from build123d import *

# Parameters (mm, degrees)
SKETCH_1_W               = 45
SKETCH_1_H               = 45
EXTRUDE_1_DEPTH          = 2.5
EXTRUDE_2_DEPTH          = 50
SKETCH_3_R               = 5.5
CUT_EXTRUDE_1_DEPTH      = 80.633535649
CUT_EXTRUDE_2_DEPTH      = 80.633535649
SKETCH_5_W               = 5
SKETCH_5_H               = 39.075696326
EXTRUDE_3_DEPTH          = 10
CUT_EXTRUDE_3_DEPTH      = 81.922374398
SKETCH_7_W               = 5.5
SKETCH_7_H               = 39.075696326
EXTRUDE_4_DEPTH          = 20
CUT_EXTRUDE_4_DEPTH      = 83.5
CUT_EXTRUDE_5_DEPTH      = 81.922374398
CUT_EXTRUDE_7_REACH      = 84.5
SKETCH_12_R              = 1.5
SKETCH_12_R_2            = 1.525256865
SKETCH_12_R_3            = 1.450491537
CUT_EXTRUDE_8_DEPTH      = 10
CUT_EXTRUDE_8_DEPTH_BACK = 0.001
SKETCH_13_R              = 2.5


with BuildPart() as part:
    # 草图1 → 凸台-拉伸1 (new body)
    with BuildSketch(Plane.XY):
        with Locations((22.5, 22.5)):
            Rectangle(SKETCH_1_W, SKETCH_1_H)
    extrude(amount=EXTRUDE_1_DEPTH)

    # 草图2 → 凸台-拉伸2 (add)
    with BuildSketch(Plane.XY.offset(2.5)):
        Polygon((36.5, 22.5), (36.5, 0), (39.5, 0), (39.5, 45), (36.5, 45), align=None)
        Polygon((8.5, 45), (8.5, 22.5), (8.5, 0), (5.5, 0), (5.5, 45), align=None)
    extrude(amount=EXTRUDE_2_DEPTH)

    # 草图3 → 切除-拉伸1 (cut, through all)
    with BuildSketch(Plane(origin=(39.5, 0, 0), x_dir=(0, 0, -1), z_dir=(1, 0, 0))):
        with Locations((-42, 22.5)):
            Circle(SKETCH_3_R)
    extrude(amount=-CUT_EXTRUDE_1_DEPTH, mode=Mode.SUBTRACT)

    # 草图4 → 切除-拉伸2 (cut, through all)
    with BuildSketch(Plane(origin=(39.5, 0, 0), x_dir=(0, 0, -1), z_dir=(1, 0, 0))):
        with BuildLine():
            Line((-2.5, 45), (-2.5, 41.474247654))
            ThreePointArc((-2.5, 41.474247654), (-25.225749209, 40.564939101), (-46.358725725, 32.157571933))
            ThreePointArc((-46.358725725, 32.157571933), (-50.832231318, 28.283182945), (-52.5, 22.605006306))
            Line((-52.5, 22.605006306), (-52.5, 45))
            Line((-52.5, 45), (-2.5, 45))
        make_face()
        with BuildLine():
            Line((-52.5, 22.394993694), (-52.5, 0))
            Line((-52.5, 0), (-2.5, 0))
            Line((-2.5, 0), (-2.5, 3.525752346))
            ThreePointArc((-2.5, 3.525752346), (-25.225749209, 4.435060899), (-46.358725725, 12.842428067))
            ThreePointArc((-46.358725725, 12.842428067), (-50.832231318, 16.716817055), (-52.5, 22.394993694))
        make_face()
    extrude(amount=-CUT_EXTRUDE_2_DEPTH, mode=Mode.SUBTRACT)

    # 草图5 → 凸台-拉伸3 (add)
    with BuildSketch(Plane.XY.offset(2.5)):
        with Locations((11, 22.5)):
            Rectangle(SKETCH_5_W, SKETCH_5_H)
        with Locations((34, 22.5)):
            Rectangle(SKETCH_5_W, SKETCH_5_H)
    extrude(amount=EXTRUDE_3_DEPTH)

    # 草图6 → 切除-拉伸3 (cut, through all)
    with BuildSketch(Plane(origin=(0, 42.037848163, 0), x_dir=(1, 0, 0), z_dir=(0, 1, 0))):
        with BuildLine():
            Line((13.5, -2.5), (13.5, -12.5))
            Line((13.5, -12.5), (8.5, -12.5))
            ThreePointArc((8.5, -12.5), (9.861833326, -6.930916663), (13.5, -2.5))
        make_face()
        with BuildLine():
            Line((31.5, -2.5), (31.5, -12.5))
            Line((31.5, -12.5), (36.5, -12.5))
            ThreePointArc((36.5, -12.5), (35.138166674, -6.930916663), (31.5, -2.5))
        make_face()
    extrude(amount=-CUT_EXTRUDE_3_DEPTH, mode=Mode.SUBTRACT)

    # 草图7 → 凸台-拉伸4 (add)
    with BuildSketch(Plane.XY.offset(2.5)):
        with Locations((2.75, 22.5)):
            Rectangle(SKETCH_7_W, SKETCH_7_H)
        with Locations((42.25, 22.5)):
            Rectangle(SKETCH_7_W, SKETCH_7_H)
    extrude(amount=EXTRUDE_4_DEPTH)

    # 草图8 → 切除-拉伸4 (cut, through all)
    with BuildSketch(Plane(origin=(45, 0, 0), x_dir=(0, 0, -1), z_dir=(1, 0, 0))):
        with BuildLine():
            Line((-22.5, 41.085625399), (-22.5, 42.037848163))
            Line((-22.5, 42.037848163), (-17.008220021, 42.037848163))
            ThreePointArc((-17.008220021, 42.037848163), (-19.771631621, 41.662789638), (-22.5, 41.085625399))
        make_face()
        with BuildLine():
            Line((-22.5, 3.914374601), (-22.5, 2.962151837))
            Line((-22.5, 2.962151837), (-17.008220021, 2.962151837))
            ThreePointArc((-17.008220021, 2.962151837), (-19.771631621, 3.337210362), (-22.5, 3.914374601))
        make_face()
    extrude(amount=-CUT_EXTRUDE_4_DEPTH, mode=Mode.SUBTRACT)

    # 草图9 → 切除-拉伸5 (cut, through all)
    with BuildSketch(Plane(origin=(0, 2.962151837, 0), x_dir=(-1, 0, 0), z_dir=(0, -1, 0))):
        with BuildLine():
            Line((-39.5, -22.5), (-45, -22.5))
            Line((-45, -22.5), (-45, -2.5))
            ThreePointArc((-45, -2.5), (-41.339785895, -12.249691121), (-39.5, -22.5))
        make_face()
        with BuildLine():
            Line((-5.5, -22.5), (0, -22.5))
            Line((0, -22.5), (0, -2.5))
            ThreePointArc((0, -2.5), (-3.660214105, -12.249691121), (-5.5, -22.5))
        make_face()
    extrude(amount=-CUT_EXTRUDE_5_DEPTH, mode=Mode.SUBTRACT)

    # 草图12 → 切除-拉伸7 (cut, up to next)
    with BuildSketch(Plane(origin=(0, 0, 0), x_dir=(-1, 0, 0), z_dir=(0, 0, -1)), mode=Mode.PRIVATE) as cut_extrude_7_sk1:
        with Locations((-13.5, 18.5)):
            Circle(SKETCH_12_R)
    cut_extrude_7_tool1 = extrude(cut_extrude_7_sk1.sketch, amount=-CUT_EXTRUDE_7_REACH, mode=Mode.PRIVATE) & part.part
    # 草图12 → 切除-拉伸7 (cut, up to next)
    with BuildSketch(Plane(origin=(0, 0, 0), x_dir=(-1, 0, 0), z_dir=(0, 0, -1)), mode=Mode.PRIVATE) as cut_extrude_7_sk2:
        with Locations((-13.5, 6.5)):
            Circle(SKETCH_12_R_2)
    cut_extrude_7_tool2 = extrude(cut_extrude_7_sk2.sketch, amount=-CUT_EXTRUDE_7_REACH, mode=Mode.PRIVATE) & part.part
    # 草图12 → 切除-拉伸7 (cut, up to next)
    with BuildSketch(Plane(origin=(0, 0, 0), x_dir=(-1, 0, 0), z_dir=(0, 0, -1)), mode=Mode.PRIVATE) as cut_extrude_7_sk3:
        with Locations((-31.5, 18.5)):
            Circle(SKETCH_12_R)
    cut_extrude_7_tool3 = extrude(cut_extrude_7_sk3.sketch, amount=-CUT_EXTRUDE_7_REACH, mode=Mode.PRIVATE) & part.part
    # 草图12 → 切除-拉伸7 (cut, up to next)
    with BuildSketch(Plane(origin=(0, 0, 0), x_dir=(-1, 0, 0), z_dir=(0, 0, -1)), mode=Mode.PRIVATE) as cut_extrude_7_sk4:
        with Locations((-31.5, 6.5)):
            Circle(SKETCH_12_R_3)
    cut_extrude_7_tool4 = extrude(cut_extrude_7_sk4.sketch, amount=-CUT_EXTRUDE_7_REACH, mode=Mode.PRIVATE) & part.part
    # 草图12 → 切除-拉伸7 (cut, up to next)
    with BuildSketch(Plane(origin=(0, 0, 0), x_dir=(-1, 0, 0), z_dir=(0, 0, -1)), mode=Mode.PRIVATE) as cut_extrude_7_sk5:
        with Locations((-13.5, 41)):
            Circle(SKETCH_12_R)
    cut_extrude_7_tool5 = extrude(cut_extrude_7_sk5.sketch, amount=-CUT_EXTRUDE_7_REACH, mode=Mode.PRIVATE) & part.part
    # 草图12 → 切除-拉伸7 (cut, up to next)
    with BuildSketch(Plane(origin=(0, 0, 0), x_dir=(-1, 0, 0), z_dir=(0, 0, -1)), mode=Mode.PRIVATE) as cut_extrude_7_sk6:
        with Locations((-31.5, 41)):
            Circle(SKETCH_12_R)
    cut_extrude_7_tool6 = extrude(cut_extrude_7_sk6.sketch, amount=-CUT_EXTRUDE_7_REACH, mode=Mode.PRIVATE) & part.part
    # 草图12 → 切除-拉伸7 (cut, up to next)
    with BuildSketch(Plane(origin=(0, 0, 0), x_dir=(-1, 0, 0), z_dir=(0, 0, -1)), mode=Mode.PRIVATE) as cut_extrude_7_sk7:
        with Locations((-22.5, 29.75)):
            Circle(SKETCH_12_R)
    cut_extrude_7_tool7 = extrude(cut_extrude_7_sk7.sketch, amount=-CUT_EXTRUDE_7_REACH, mode=Mode.PRIVATE) & part.part
    add(cut_extrude_7_tool1.solids().sort_by_distance((13.5, 18.5, 0))[0], mode=Mode.SUBTRACT)
    add(cut_extrude_7_tool2.solids().sort_by_distance((13.5, 6.5, 0))[0], mode=Mode.SUBTRACT)
    add(cut_extrude_7_tool3.solids().sort_by_distance((31.5, 18.5, 0))[0], mode=Mode.SUBTRACT)
    add(cut_extrude_7_tool4.solids().sort_by_distance((31.5, 6.5, 0))[0], mode=Mode.SUBTRACT)
    add(cut_extrude_7_tool5.solids().sort_by_distance((13.5, 41, 0))[0], mode=Mode.SUBTRACT)
    add(cut_extrude_7_tool6.solids().sort_by_distance((31.5, 41, 0))[0], mode=Mode.SUBTRACT)
    add(cut_extrude_7_tool7.solids().sort_by_distance((22.5, 29.75, 0))[0], mode=Mode.SUBTRACT)

    # 草图13 → 切除-拉伸8 (cut, two sides: drawn at the far end of the back side and taken through both)
    with BuildSketch(Plane.XY.offset(2.5).offset(-CUT_EXTRUDE_8_DEPTH_BACK)):
        with Locations(Location((13.5, 6.5, 0), (0, 0, 180))):
            Circle(SKETCH_13_R)
        with Locations(Location((13.5, 18.5, 0), (0, 0, 180))):
            Circle(SKETCH_13_R)
        with Locations(Location((13.5, 41, 0), (0, 0, 180))):
            Circle(SKETCH_13_R)
        with Locations(Location((31.5, 41, 0), (0, 0, 180))):
            Circle(SKETCH_13_R)
        with Locations(Location((31.5, 18.5, 0), (0, 0, 180))):
            Circle(SKETCH_13_R)
        with Locations(Location((31.5, 6.5, 0), (0, 0, 180))):
            Circle(SKETCH_13_R)
    extrude(amount=CUT_EXTRUDE_8_DEPTH + CUT_EXTRUDE_8_DEPTH_BACK, mode=Mode.SUBTRACT)


solid = part.part
Verification items for the finished model (mm, model axes). A direction names the side the tool comes from. Coordinates: 2 decimals unless noted, no trailing zeros. Loops run counter-clockwise (first coordinate to the right, second up) from the corner with the lowest first, then second, coordinate; pieces in that order, holes last. Notation, with made-up numbers: (65, -31.75) -> (114, -31.75) arc R22 cw to (114, -7.75) -> close; hole circle Ø6 at (26.25, 86.25). An arc over 180 degrees is marked (long way). Answer as CSV lines item,"result".
1) Thickness scan on L1, parallel to Y at x = 13.5, z = 1.95; L2, parallel to X at y = 20, z = 27.5; L3, parallel to Y at x = 13, z = 1. Record the ranges inside material, lowest first. Write a range as from..to.
Found:
L1,"y = 0..4.97, 8.03..17, 20..39.5, 42.5..45"
L2,"x = 5.5..8.5, 36.5..39.5"
L3,"y = 0..5.06, 7.94..17.09, 19.91..39.59, 42.41..45"
2) Cross-section at C-C, the plane y = 6.5. Count the separate pieces of the cut face and the enclosed holes in it, then the cut area to 3 significant figures.
Found:
separate pieces,"3"
enclosed holes,"0"
area,"388 mm2"
3) Release check for a two-part mould opening along X. For faces 1 (the flat face through (22, 23, 2.5)), 2 (the flat face through (45, 22, 1)), 3 (the flat face through (5.5, 22, 34)), 4 (the cylindrical face through (7.02, 16.65, 50.79)) record: +X half, -X half, draft (parallel to the pull), parting line (faces both ways), or undercut.
Found:
face 1,"undercut"
face 2,"+X half"
face 3,"-X half"
face 4,"draft"
4) Cross-section at A-A, the plane z = 16. Record the cut outline in (x, y).
Found:
outline,"(4.56, 2.96) -> (5.5, 2.96) -> (5.5, 3.13) -> (8.5, 3.13) -> (8.5, 41.87) -> (5.5, 41.87) -> (5.5, 42.04) -> (4.56, 42.04) -> close; (36.5, 3.13) -> (39.5, 3.13) -> (39.5, 2.96) -> (40.44, 2.96) -> (40.44, 42.04) -> (39.5, 42.04) -> (39.5, 41.87) -> (36.5, 41.87) -> close"
5) Cross-section at D-D, the plane y = 14. Record the cut outline in (x, z).
Found:
outline,"(0, 0) -> (45, 0) -> (45, 2.5) arc R57.44 cw to (39.5, 22.5) -> (39.5, 48.31) -> (36.5, 48.31) -> (36.5, 12.5) arc R12.92 cw to (31.5, 2.5) -> (13.5, 2.5) arc R12.92 cw to (8.5, 12.5) -> (8.5, 48.31) -> (5.5, 48.31) -> (5.5, 22.5) arc R57.44 cw to (0, 2.5) -> close"
6) Tool access check on faces 5 (the flat face through (35, 2.962, 5)), 6 (the flat face through (30, 20, 2.499)), 7 (the flat face through (36.5, 23, 28)). Record the directions out of +Z, -Z, +X, -X, +Y, -Y that give a thin tool (end or side, any length) a straight path to the whole face; none if there is none.
Found:
face 5,"+Z, +X, -X, -Y"
face 6,"+Z"
face 7,"+Z, +Y, -Y"
7) Depth check by flat-ended pin: pin 1 (0.6 mm diameter, centred on y = 42, z = 9, fed in from -X); pin 2 (5 mm diameter, centred on y = 26, z = 11.5, fed in from +X); pin 3 (1 mm diameter, centred on y = 3.5, z = 16.5, fed in from +X); pin 4 (2.5 mm diameter, centred on x = 31.5, y = 41, fed in from +Z). Enter the tip coordinate at first touch or a pass-through.
Found:
pin 1,"stops at x = 2.56"
pin 2,"stops at x = 42.34"
pin 3,"stops at x = 40.44"
pin 4,"passes through"
8) Cross-section at B-B, the plane z = 44.5. Record the cut outline in (x, y), then the cut area to 3 significant figures.
Found:
outline,"(5.5, 11.75) -> (8.5, 11.75) -> (8.5, 17.6) -> (5.5, 17.6) -> close; (5.5, 27.4) -> (8.5, 27.4) -> (8.5, 33.25) -> (5.5, 33.25) -> close; (36.5, 11.75) -> (39.5, 11.75) -> (39.5, 17.6) -> (36.5, 17.6) -> close; (36.5, 27.4) -> (39.5, 27.4) -> (39.5, 33.25) -> (36.5, 33.25) -> close"
area,"70.2 mm2"
